CAD build for the part. Positions are in the model's coordinates, mm. A direction names the side the tool comes from. Give positions to 0.01 mm unless a question says otherwise; leave off trailing zeros. Loops run counter-clockwise (first coordinate to the right, second up) from the corner with the lowest first, then second, coordinate; pieces in that order, holes last. Notation, with made-up numbers: M 5,-39 L 34,-39 A32 ccw 34,-6 Z; hole C 51.25,84 d11. An arc over 180 degrees is marked long. Answer as CSV lines item,"result".
Autodesk Inventor part; units mm, degrees
ref_plane "YZ Plane" through (0, 0, 0) normal (1, 0, 0) x (0, 1, 0)
ref_plane "XZ Plane" through (0, 0, 0) normal (0, 1, 0) x (-1, 0, 0)
ref_plane "XY Plane" through (0, 0, 0) normal (0, 0, 1) x (1, 0, 0)
sketch "Sketch1" plane through (0, 0, 0) normal (0, 1, 0) x (-1, 0, 0)
  line L0 (100, 125) -> (-100, 125)
  line L1 (-100, 125) -> (-100, -125)
  line L2 (-100, -125) -> (100, -125)
  line L3 (100, -125) -> (100, 125)
  line L4 (100, 125) -> (-100, -125) construction
  line L5 (-100, 125) -> (100, -125) construction
  circle A0 centre (0, 12.655) radius 8.2
  circle A1 centre (0, -12.655) radius 8.2
  line L6 (10.65, 6) -> (6.0435, 6)
  line L7 (6.0435, 6) -> (6.0435, -6)
  line L8 (6.0435, -6) -> (10.65, -6)
  line L9 (10.65, -6) -> (10.65, 6)
  line L10 (10.65, 6) -> (6.0435, -6) construction
  line L11 (6.0435, 6) -> (10.65, -6) construction
  circle A2 centre (0, -117) radius 1.875
  circle A3 centre (-25.8, -117) radius 1.875
  circle A4 centre (25.8, -117) radius 1.875
  point P0 (0, 0)
  dimension "d0" = 200
  dimension "d1" = 250
  dimension "d2" = 16.4
  dimension "d3" = 16.4
  dimension "d7" = 4.6065
  dimension "d8" = 12
  dimension "d14" = 3.75
  dimension "d15" = 3.75
  dimension "d16" = 3.75
  dimension "d17" = 8
  dimension "d18" = 8
  dimension "d19" = 8
  dimension "d20" = 25.8
  dimension "d21" = 25.8
extrude "Extrusion1" add sketch "Sketch1" along normal blind 3
sketch "Sketch2" plane through (0, 3, 0) normal (0, 1, 0) x (1, 0, 0)
  line L0 (-20, 25) -> (20, 25)
  line L1 (20, 25) -> (20, -25)
  line L2 (20, -25) -> (-20, -25)
  line L3 (-20, -25) -> (-20, 25)
  line L4 (-20, 25) -> (20, -25) construction
  line L5 (20, 25) -> (-20, -25) construction
  line L6 (-23, 28) -> (23, 28)
  line L7 (23, 28) -> (23, -28)
  line L8 (23, -28) -> (-23, -28)
  line L9 (-23, -28) -> (-23, 28)
  line L10 (-23, 28) -> (23, -28) construction
  line L11 (23, 28) -> (-23, -28) construction
  point P0 (0, 0)
  dimension "d24" = 40
  dimension "d25" = 50
  dimension "d26" = 46
  dimension "d27" = 56
extrude "Extrusion2" add sketch "Sketch2" along normal blind 37
sketch "Sketch3" plane through (0, 40, 0) normal (0, 1, 0) x (1, 0, 0)
  line L0 (-23, -28) -> (23, -28)
  line L1 (-23, 28) -> (23, 28)
  line L2 (23, 28) -> (23, -28)
  line L3 (23, -28) -> (-23, -28)
  line L4 (-23, -28) -> (-23, 28)
  line L5 (-23, 28) -> (23, -28) construction
  line L6 (23, 28) -> (-23, -28) construction
  point P0 (0, 0)
extrude "Extrusion3" add sketch "Sketch3" along normal blind 3
fillet "Fillet1" radius 2 8 edges at (0, 43, 28) (23, 43, 0) (0, 43, -28) (-23, 43, 0) (-23, 23, 28) (23, 23, 28) (23, 23, -28) (-23, 23, -28)
properties part number "top_sensor"
1) Band-saw the part on C-C on z = 86. Give the cut face in (x, y), and give its area (3 significant figures).
Answer below:
outline,"M -100,0 L 100,0 L 100,3 L -100,3 Z"
area,"600 mm^2"
2) Drill centre lines: line 1 (X direction, y = 2.25, z = -117) (3 decimals); line 2 (Z direction, x = 0, y = 1) (3 decimals); line 3 (Z direction, x = 1, y = 25). Where is each one in solid material? Low to high. Write a range as from..to.
Answer below:
line 1,"x = -100..-27.675, -23.925..-1.875, 1.875..23.925, 27.675..100"
line 2,"z = -125..-118.875, -115.125..-20.855, -4.455..4.455, 20.855..125"
line 3,"z = -28..-25, 25..28"
3) Flat gauge pins, fed straight in: pin 1 (6 mm diameter, centred on x = 0, z = -117, fed in from +Y); pin 2 (19 mm diameter, centred on x = -6.5, y = 31.5, fed in from -Z); pin 3 (11.5 mm diameter, centred on x = -10, y = 23, fed in from +Z). Where does each tip first touch, or does it go through?
Answer below:
pin 1,"stops at y = 3"
pin 2,"stops at z = -28"
pin 3,"stops at z = 28"
4) Band-saw the part on B-B on y = 24.5. Give the cut face in (x, z), and give its area (3 significant figures).
Answer below:
outline,"M -23,-26 A2 ccw -21,-28 L 21,-28 A2 ccw 23,-26 L 23,26 A2 ccw 21,28 L -21,28 A2 ccw -23,26 Z; hole M -20,-25 L 20,-25 L 20,25 L -20,25 Z"
area,"573 mm^2"
5) Band-saw the part on A-A on x = -15. Give the cut face in (y, z).
Answer below:
outline,"M 0,-125 L 3,-125 L 3,-28 L 41,-28 A2 ccw 43,-26 L 43,26 A2 ccw 41,28 L 3,28 L 3,125 L 0,125 Z; hole M 3,-25 L 40,-25 L 40,25 L 3,25 Z"
6) Which spindle directions (+Z, -Z, +X, -X, +Y, -Y) get a long thin tool onto all of the face, cutting with end or side? Do faces 4 (the face through (-23, 22, 0)), 5 (the face through (0, 3, 0)), 6 (the face through (0, 22, 28)), 7 (the face through (23, 22, 0)). Say none if no direction does.
Answer below:
face 4,"+Z, -Z, -X, +Y"
face 5,"none"
face 6,"+Z, +X, -X, +Y"
face 7,"+Z, -Z, +X, +Y"
7) Mould opens along Y. For faces 1 (the face through (20, 21, 0)), 2 (the face through (1.78, 1.48, 20.66)), 3 (the face through (1, 0, 2)) say: +Y half, -Y half, draft (parallel to the pull), parting line (faces both ways), or undercut.
Answer below:
face 1,"undercut"
face 2,"draft"
face 3,"-Y half"
8) Band-saw the part on D-D on x = 69.5. Give the cut face in (y, z), and give its area (3 significant figures).
Answer below:
outline,"M 0,-125 L 3,-125 L 3,125 L 0,125 Z"
area,"750 mm^2"
